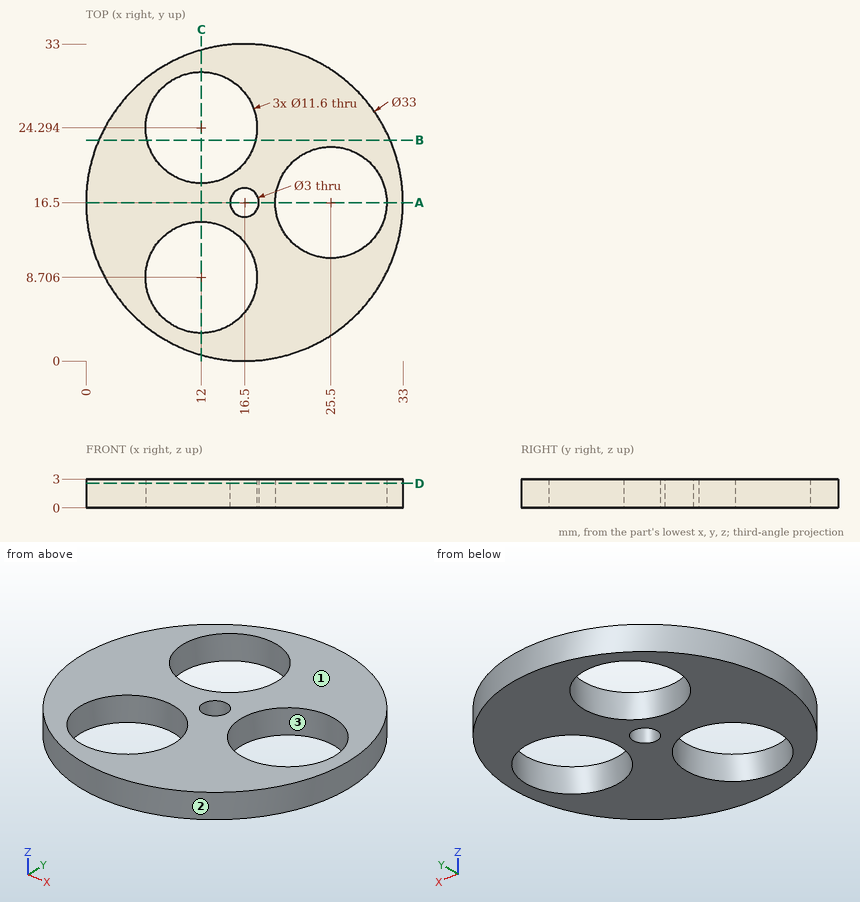
Can you work these out from the drawing? Everything is in mm from the part's minimum corner. Give positions to 0.01 mm unless a question says otherwise; leave off trailing zeros. Order: outer loops, then holes, each group sorted by start corner. A loop starts at its lowest first (then second) coordinate and runs counter-clockwise, first axis right, second up. Notation, with made-up numbers: M 24.5,-22 L 41.5,-22 A15 ccw 41.5,1 Z; hole C 57,-39 d11. An arc over 180 degrees is marked long. Use a Markdown table: item, result. Add a question column.
Item 1: Suppose I cut it at C-C (x = 12). List the corners of the cut face in (y, z) for me.
Item 2: If I drill on L1, parallel to Y at x = 16.5, z = 2.25 (1 decimal); L2, parallel to X at y = 12, z = 2.2 (1 decimal); L3, parallel to X at y = 19.5, z = 1.55 (1 decimal), over which ranges is the centre line in solid material (lowest first)? Write a range as [from, to].
Item 3: Will these pins go through, and if not, where does the flat tip stop? pin 1 (1.5 mm diameter, centred on y = 15.5, z = 2, fed in from +X); pin 2 (1 mm diameter, centred on y = 6.5, z = 1.5, fed in from -X); pin 3 (1 mm diameter, centred on x = 18, z = 2, fed in from -Y).
Item 4: Suppose I cut it at A-A (y = 16.5). List the corners of the cut face in (x, z) for me.
Item 5: We'd pull the mould along Y, two halves only. Please class the marked faces 1, 2 and 3: +Y half, -Y half, draft (parallel to the pull), parting line (faces both ways), or undercut.
Item 6: Suppose I cut it at D-D (z = 2.55). List the corners of the cut face in (x, y) for me, then the cut area to 3 significant figures.
Item 7: Suppose I cut it at B-B (y = 23). List the corners of the cut face in (x, z) for me.
Answer sheet:
| question | item | result |
|---|---|---|
| 1 | outline | M 0.63,0 L 2.91,0 L 2.91,3 L 0.63,3 Z; M 14.51,0 L 18.49,0 L 18.49,3 L 14.51,3 Z; M 30.09,0 L 32.37,0 L 32.37,3 L 30.09,3 Z |
| 2 | L1 | y = [0, 5], [12.4, 15], [18, 20.6], [28, 33] |
| 2 | L2 | x = [0.6, 7.2], [16.8, 21.8], [29.2, 32.4] |
| 2 | L3 | x = [0.3, 8.7], [15.3, 20.5], [30.5, 32.7] |
| 3 | pin 1 | stops at x = 33 |
| 3 | pin 2 | stops at x = 3.01 |
| 3 | pin 3 | stops at y = 0.03 |
| 4 | outline | M 0,0 L 15,0 L 15,3 L 0,3 Z; M 18,0 L 19.7,0 L 19.7,3 L 18,3 Z; M 31.3,0 L 33,0 L 33,3 L 31.3,3 Z |
| 5 | face 1 | draft |
| 5 | face 2 | parting line |
| 5 | face 3 | undercut |
| 6 | outline | C 16.5,16.5 d33; hole C 12,8.71 d11.6; hole C 12,24.29 d11.6; hole C 16.5,16.5 d3; hole C 25.5,16.5 d11.6 |
| 6 | area | 531 mm² |
| 7 | outline | M 1.33,0 L 6.35,0 L 6.35,3 L 1.33,3 Z; M 17.65,0 L 31.67,0 L 31.67,3 L 17.65,3 Z |
